```python
from build123d import *

# Parameters (mm, degrees)
F1_DEPTH = 250


with BuildPart() as f1:
    # F0 (on Top) → F1 (new body)
    with BuildSketch(Plane.XY):
        with BuildLine():
            Line((-54, 0), (0, 0))
            Line((0, 0), (0, 4.5))
            Line((0, 4.5), (-49.5, 4.5))
            ThreePointArc((-49.5, 4.5), (-53.742641, 6.257359), (-55.5, 10.5))
            Line((-55.5, 10.5), (-55.5, 130.388169))
            ThreePointArc((-55.5, 130.388169), (-53.925689, 134.439499), (-50.028906, 136.364811))
            Line((-50.028906, 136.364811), (41.971094, 144.506404))
            ThreePointArc((41.971094, 144.506404), (46.551331, 142.95545), (48.5, 138.529761))
            Line((48.5, 138.529761), (48.5, 123.5))
            ThreePointArc((48.5, 123.5), (50.257359, 119.257359), (54.5, 117.5))
            Line((54.5, 117.5), (98, 117.5))
            Line((98, 117.5), (98, 122))
            Line((98, 122), (59, 122))
            ThreePointArc((59, 122), (54.757359, 123.757359), (53, 128))
            Line((53, 128), (53, 143.445578))
            ThreePointArc((53, 143.445578), (51.051331, 147.871267), (46.471094, 149.422221))
            Line((46.471094, 149.422221), (-54.528906, 140.484168))
            ThreePointArc((-54.528906, 140.484168), (-58.425689, 138.558856), (-60, 134.507525))
            Line((-60, 134.507525), (-60, 6))
            ThreePointArc((-60, 6), (-58.242641, 1.757359), (-54, 0))
        make_face()
    extrude(amount=F1_DEPTH)


solid = f1.part
```
Could you check a few things on this model? Use its own coordinates, in mm. A direction names the side the tool comes from. Round coordinates to 2 decimals unless told otherwise and drop trailing zeros. Loops run counter-clockwise (first coordinate to the right, second up) from the corner with the lowest first, then second, coordinate; pieces in that order, holes last. Notation, with made-up numbers: M -16,55 L 13,55 A35 cw 13,93 Z; hole C -12.75,-3 d4. An arc over 180 degrees is marked long. Put each result on its own line as item: value.
Q1. Thinking about a two-plate mould opening in Y: for faces 4 (the face through (-55.5, 70, 123)), 5 (the face through (48.5, 131, 123)), 6 (the face through (50.211, 119.304, 123.25)), which applies, released by +Y, released by -Y, zero draft, split by the parting line, or undercut?
Check result:
face 4: undercut
face 5: zero draft
face 6: released by -Y
Q2. Imagine slicing it at B-B (x = -18). Write out the boundary of the cut face in (y, z), then the cut area to 3 significant figures.
Check result:
outline: M 0,0 L 4.5,0 L 4.5,250 L 0,250 Z; M 139.2,0 L 143.72,0 L 143.72,250 L 139.2,250 Z
area: 2,250 mm2
Q3. I need wall thicknesses on probe 1 along Y at (x, z) = (68.5, 173); probe 2 along X at (y, z) = (66, 32.5); probe 3 along X at (y, z) = (119, 47). Which ranges of each line are inside material? Lowest first, please.
Check result:
probe 1: 117.5 to 122
probe 2: -60 to -55.5
probe 3: -60 to -55.5, 50.53 to 98
Q4. Imagine slicing it at D-D (x = 22.5). Write out the boundary of the cut face in (y, z), then the cut area to 3 significant figures.
Check result:
outline: M 142.78,0 L 147.3,0 L 147.3,250 L 142.78,250 Z
area: 1,130 mm2
Q5. On a 3-axis mill with a long thin cutter (end or side, diameter ignored), from which of +Z, -Z, +X, -X, +Y, -Y can I reach the whole of each face in a straight line? I mean faces 1 (the face through (-4.67, 140.38, 123.25)), 2 (the face through (76, 117.5, 123)), 3 (the face through (-24, 4.5, 123)). Say none if no direction works.
Check result:
face 1: +Z, -Z
face 2: +Z, -Z, +X, -Y
face 3: +Z, -Z, +X
Q6. Imagine slicing it at C-C (y = 92.5). Write out the boundary of the cut face in (x, z).
Check result:
outline: M -60,0 L -55.5,0 L -55.5,250 L -60,250 Z
Q7. For pin 1 (12 mm diameter, centred on x = -34, z = 31, fed in from +Y); pin 2 (22 mm diameter, centred on x = 69, z = 162.5, fed in from -Y); pin 3 (6 mm diameter, centred on x = -9, z = 148.5, fed in from +Y), each with a flat end and sliding along its axis, tell me the tip position at first contact or that it passes through.
Check result:
pin 1: y = 142.83
pin 2: y = 117.5
pin 3: y = 144.78
Q8. Imagine slicing it at A-A (z = 48). Write out the boundary of the cut face in (x, y), then the cut area to 3 significant figures.
Check result:
outline: M -60,6 A6 ccw -54,0 L 0,0 L 0,4.5 L -49.5,4.5 A6 cw -55.5,10.5 L -55.5,130.39 A6 cw -50.03,136.36 L 41.97,144.51 A6 cw 48.5,138.53 L 48.5,123.5 A6 ccw 54.5,117.5 L 98,117.5 L 98,122 L 59,122 A6 cw 53,128 L 53,143.45 A6 ccw 46.47,149.42 L -54.53,140.48 A6 ccw -60,134.51 Z
area: 1,700 mm2
